from build123d import *

# Parameters (mm, degrees)
SKETCH_2_R   = 5
SKETCH_2_R_2 = 4


with BuildPart() as part:
    # По траектории1: sweep along a path in Эскиз1
    with BuildLine(Plane(origin=(0, 0, 0), x_dir=(1, 0, 0), z_dir=(0, 1, 0))) as sweep_1_path:
        Line((0, 0), (20, 0))
        ThreePointArc((20, 0), (27.071067812, 2.928932188), (30, 10))
        Line((30, 10), (30, 120))
    # Эскиз2 → По траектории1 (sweep)
    with BuildSketch(Plane(origin=(0, 0, 0), x_dir=(0, 0, -1), z_dir=(1, 0, 0))):
        Circle(SKETCH_2_R)
        Circle(SKETCH_2_R_2, mode=Mode.SUBTRACT)
    sweep(path=sweep_1_path.line)

    # Эскиз3 → Повернуть1 (revolve)
    with BuildSketch(Plane.XY, mode=Mode.PRIVATE) as revolve_1_sk:
        Polygon((0, 7), (0, 4), (4, 4), (4, 5), align=None)
    revolve(revolve_1_sk.sketch.rotate(Axis((-3.453428096, 0, 0), (1, 0, 0)), 90), axis=Axis((-3.453428096, 0, 0), (1, 0, 0)))


solid = part.part
Build history of the part. All positions in model axes, mm. A direction names the side the tool comes from. Coordinates: 2 decimals unless noted, no trailing zeros. Write each loop counter-clockwise with the first axis right and the second up, starting at its lowest first coordinate (ties: lowest second). Pieces come first, ordered by that corner, then holes. Notation, with made-up numbers: (-32.5, 76.5) -> (16.5, 76.5) arc R11 ccw to (16.5, 92.5) -> close; hole circle Ø7 at (17.5, 33.5). An arc over 180 degrees is marked (long way). Use CSV: the item, a comma, the result in double quotes. Start each with the question number.
Q1. Cut at B-B, the plane z = -55. List the corners of the cut face in (x, y), then the cut area to 3 significant figures.
Q2. 3-axis set-ups, long thin cutter, end or side, ignore diameter. For faces 1 (the conical face through (3.75, 5.003, -1.111)), 2 (the cylindrical face through (30.867, -3.905, -65.77)): which of +Z, -Z, +X, -X, +Y, -Y reach the whole face in a straight line?
Q3. Drill centre lines: probe 1 along Y at (x, z) = (30, -43.5); probe 2 along Z at (x, y) = (11, -0.25); probe 3 along X at (y, z) = (0.25, -29.5). Where is each one in solid material? Low to high.
Q4. Pull direction X, two halves, no side cores. Call faces 3 (the flat face through (0, 3, 3)), 4 (the cylindrical face through (12.11, -4.88, 1.08)), 5 (the cylindrical face through (10.14, -3.905, 0.867)): released by +X, released by -X, zero draft, split by the parting line, or undercut.
Q5. Flat gauge pins, fed straight in: pin 1 Ø2 at (x, y) = (26, -3) entering from +Z; pin 2 Ø5 at (x, y) = (30, 0) entering from +Z; pin 3 Ø12 at (x, z) = (22, -31.5) entering from -Y. Where does each tip first touch, or does it go through?
Q6. Cut at A-A, the plane y = 0. List the corners of the cut face in (x, z).
Checked values:
1,outline,"circle Ø10 at (30, 0); hole circle Ø8 at (30, 0)"
1,area,"28.3 mm²"
2,face 1,"none"
2,face 2,"-Z"
3,probe 1,"y = -5 to -4, 4 to 5"
3,probe 2,"z = -4.99 to -3.99, 3.99 to 4.99"
3,probe 3,"x = 25.01 to 26.01, 33.99 to 34.99"
4,face 3,"released by -X"
4,face 4,"undercut"
4,face 5,"zero draft"
5,pin 1,"stops at z = 3.45"
5,pin 2,"stops at z = 2.99"
5,pin 3,"stops at y = -4.58"
6,outline,"(0, -7) -> (4, -5) -> (20, -5) arc R5 cw to (25, -10) -> (25, -120) -> (26, -120) -> (26, -10) arc R6 ccw to (20, -4) -> (0, -4) -> close; (0, 4) -> (20, 4) arc R14 cw to (34, -10) -> (34, -120) -> (35, -120) -> (35, -10) arc R15 ccw to (20, 5) -> (4, 5) -> (0, 7) -> close"
